from build123d import *
from build123d.topology import SkipClean

# Parameters (mm, degrees)
SKETCH1_R           = 50
SKETCH1_R_2         = 6
BOSS_EXTRUDE1_DEPTH = 15
SKETCH2_R           = 25
SKETCH2_R_2         = 15
BOSS_EXTRUDE2_DEPTH = 70
BOSS_EXTRUDE3_DEPTH = 15
CUT_EXTRUDE1_START  = -40
SKETCH4_R           = 15
SKETCH4_R_2         = 5
CUT_EXTRUDE1_DEPTH  = 40


with BuildPart() as part:
    # Sketch1 → Boss-Extrude1 (new body)
    with BuildSketch(Plane(origin=(0, 0, 0), x_dir=(1, 0, 0), z_dir=(0, 1, 0))):
        with Locations(Location((0, 0, 0), (0, 0, 270))):
            Circle(SKETCH1_R)
        with Locations(Location((-35, 0, 0), (0, 0, 270))):
            Circle(SKETCH1_R_2, mode=Mode.SUBTRACT)
        with Locations(Location((-17.5, 30.310889132, 0), (0, 0, 270))):
            Circle(SKETCH1_R_2, mode=Mode.SUBTRACT)
        with Locations(Location((17.5, 30.310889132, 0), (0, 0, 270))):
            Circle(SKETCH1_R_2, mode=Mode.SUBTRACT)
        with Locations(Location((35, 0, 0), (0, 0, 270))):
            Circle(SKETCH1_R_2, mode=Mode.SUBTRACT)
        with Locations(Location((17.5, -30.310889132, 0), (0, 0, 270))):
            Circle(SKETCH1_R_2, mode=Mode.SUBTRACT)
        with Locations(Location((-17.5, -30.310889132, 0), (0, 0, 270))):
            Circle(SKETCH1_R_2, mode=Mode.SUBTRACT)
    extrude(amount=BOSS_EXTRUDE1_DEPTH)

    # Sketch2 → Boss-Extrude2 (add)
    with BuildSketch(Plane(origin=(0, 15, 0), x_dir=(1, 0, 0), z_dir=(0, 1, 0))):
        with Locations(Location((0, 0, 0), (0, 0, 270))):
            Circle(SKETCH2_R)
        with Locations(Location((0, 0, 0), (0, 0, 270))):
            Circle(SKETCH2_R_2, mode=Mode.SUBTRACT)
    extrude(amount=BOSS_EXTRUDE2_DEPTH)

    # Sketch3 → Boss-Extrude3 (add)
    with SkipClean():  # the faces are left unmerged after this step: merging them gives an invalid solid
        with BuildSketch(Plane(origin=(0, 85, 0), x_dir=(1, 0, 0), z_dir=(0, 1, 0))):
            with BuildLine():
                Line((-53.125, 12.103072957), (-6.25, 24.206145914))
                ThreePointArc((-6.25, 24.206145914), (0, 25), (6.25, 24.206145914))
                Line((6.25, 24.206145914), (53.125, 12.103072957))
                ThreePointArc((53.125, 12.103072957), (62.5, 0), (53.125, -12.103072957))
                Line((53.125, -12.103072957), (6.25, -24.206145914))
                ThreePointArc((6.25, -24.206145914), (0, -25), (-6.25, -24.206145914))
                Line((-6.25, -24.206145914), (-53.125, -12.103072957))
                ThreePointArc((-53.125, -12.103072957), (-62.5, 0), (-53.125, 12.103072957))
            make_face()
        extrude(amount=BOSS_EXTRUDE3_DEPTH)

    # Sketch4 → Cut-Extrude1 (cut)
    with SkipClean():  # the faces are left unmerged after this step: merging them gives an invalid solid
        with BuildSketch(Plane(origin=(0, 100, 0), x_dir=(1, 0, 0), z_dir=(0, 1, 0)).offset(CUT_EXTRUDE1_START)):
            with Locations(Location((0, 0, 0), (0, 0, 270))):
                Circle(SKETCH4_R)
            with Locations(Location((-50, 0, 0), (0, 0, 270))):
                Circle(SKETCH4_R_2)
            with Locations(Location((50, 0, 0), (0, 0, 270))):
                Circle(SKETCH4_R_2)
        extrude(amount=CUT_EXTRUDE1_DEPTH, mode=Mode.SUBTRACT)


solid = part.part
CAD build for the part. Positions are in the model's coordinates, mm. A direction names the side the tool comes from. Round coordinates to 2 decimals unless told otherwise and drop trailing zeros. Write each loop counter-clockwise with the first axis right and the second up, starting at its lowest first coordinate (ties: lowest second). Pieces come first, ordered by that corner, then holes.
(1) Slice it at D-D, the plane z = 34. Write the cut outline in (x, y), and give its area (3 significant figures).
(2) Mould opens along X. For faces 1 (the face through (30.02, 92.4, 18.07)), 2 (the face through (54.957, 92.395, -0.651)), 3 (the face through (41, 85, 0)) say: pulls with the +X half, pulls with the -X half, needs draft (parallel to the pull), parting line crosses it, or undercut.
(3) Drop flat-ended pins along their axis: P1, Ø8, axis at y = 36.5, z = 18.5, coming from the +X side; P2, Ø6, axis at y = 70, z = -19, coming from the +X side; P3, Ø16, axis at x = -50, z = 0, coming from the +Y side; P4, Ø6, axis at y = 13.5, z = -35.5, coming from the +X side. Give the stop position or say it passes through.
(4) Slice it at A-A, the plane z = 0. Count the separate pieces of the cut face and the enclosed holes in it, and give its area (4 significant figures).
(5) 3-axis set-ups, long thin cutter, end or side, ignore diameter. For faces 4 (the face through (-45.043, 92.395, -0.651)), 5 (the face through (-40.857, 7.395, -1.301)), 6 (the face through (-29.36, 92.4, 18.24)): which of +Z, -Z, +X, -X, +Y, -Y reach the whole face in a straight line?
(6) Slice it at B-B, the plane x = 0. Write the cut outline in (y, z), and give its area (3 significant figures).
(7) Probe line 1 along X through (y, z) = (11.5, 0); line 2 along Y through (x, z) = (-26, 13); line 3 along Z through (x, y) = (1, 20.5). List the from-to ranges inside material, lowest first.
(8) Slice it at C-C, the plane y = 9.5. Write the cut outline in (x, z), and give its area (3 significant figures).
From the geometry:
1. outline: (-36.66, 0) - (-22.23, 0) - (-22.23, 15) - (-36.66, 15) - close; (-12.77, 0) - (12.77, 0) - (12.77, 15) - (-12.77, 15) - close; (22.23, 0) - (36.66, 0) - (36.66, 15) - (22.23, 15) - close
1. area: 816 mm2
2. face 1: pulls with the +X half
2. face 2: undercut
2. face 3: needs draft
3. P1: stops at x = 20.37
3. P2: stops at x = 19.21
3. P3: stops at y = 100
3. P4: stops at x = 38
4. separate pieces: 5
4. enclosed holes: 0
4. area: 3,665 mm2
5. face 4: +Y
5. face 5: -Y
5. face 6: +Z, -X, +Y
6. outline: (0, -50) - (15, -50) - (15, -25) - (100, -25) - (100, -15) - (15, -15) - (15, 15) - (100, 15) - (100, 25) - (15, 25) - (15, 50) - (0, 50) - close
6. area: 3,200 mm2
7. line 1: x = -50 to -41, -29 to 29, 41 to 50
7. line 2: y = 0 to 15, 85 to 100
7. line 3: z = -24.98 to -14.97, 14.97 to 24.98
8. outline: circle Ø100 at (0, 0); hole circle Ø12 at (-35, 0); hole circle Ø12 at (-17.5, -30.31); hole circle Ø12 at (-17.5, 30.31); hole circle Ø12 at (17.5, -30.31); hole circle Ø12 at (17.5, 30.31); hole circle Ø12 at (35, 0)
8. area: 7,180 mm2
